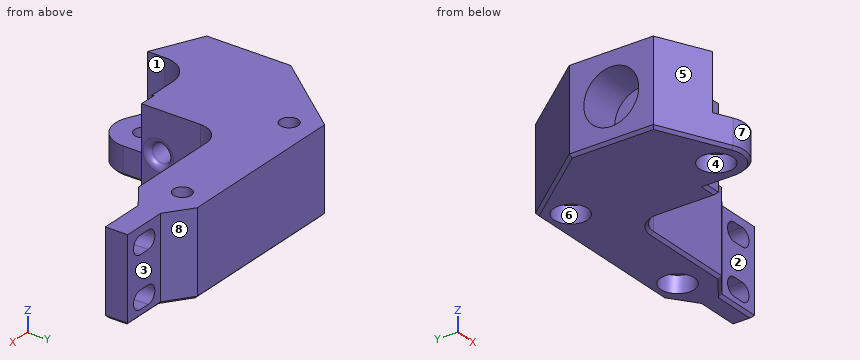
from build123d import *

# Parameters (mm, degrees)
BOX_W           = 10.4
BOX_H           = 10.4
BOX_DEPTH       = 10
CYLINDER_R      = 5.2
CYLINDER_DEPTH  = 10
BOX001_W        = 10.4
BOX001_H        = 10
BOX001_DEPTH    = 10
SKETCH001_R     = 1.6
PAD_DEPTH       = 20
SKETCH_R        = 3
PAD001_DEPTH    = 3
PAD002_DEPTH    = 15
SKETCH003_R     = 4.9
POCKET_DEPTH    = 7.5
SKETCH004_R     = 1.75
POCKET001_DEPTH = 47.501
POCKET002_DEPTH = 5
FILLET_R        = 4
FILLET001_R     = 1
CHAMFER_SIZE    = 0.5


with BuildPart() as cube:
    # Box → Box (new body)
    with BuildSketch(Plane(origin=(-13, -18.2, 5), x_dir=(1, 0, 0), z_dir=(0, 0, 1))):
        with Locations((5.2, 5.2)):
            Rectangle(BOX_W, BOX_H)
    extrude(amount=BOX_DEPTH)


with BuildPart() as cylinder:
    # Cylinder → Cylinder (new body)
    with BuildSketch(Plane(origin=(-13, -13, 5), x_dir=(1, 0, 0), z_dir=(0, 0, 1))):
        Circle(CYLINDER_R)
    extrude(amount=CYLINDER_DEPTH)


with BuildPart() as obj1:
    # Box001 → Box001 (new body)
    with BuildSketch(Plane(origin=(-18.2, -23, 5), x_dir=(1, 0, 0), z_dir=(0, 0, 1))):
        with Locations((5.2, 5)):
            Rectangle(BOX001_W, BOX001_H)
    extrude(amount=BOX001_DEPTH)

    # Fusion001: union Cube, Cylinder
    add(cube.part)
    add(cylinder.part)


with BuildPart() as cuerpo_tornillos:
    # Sketch001 → Pad (new body)
    with BuildSketch(Plane.XY.offset(3.25)):
        with Locations((-13, 13)):
            Circle(SKETCH001_R)
        with Locations((13, 13)):
            Circle(SKETCH001_R)
        with Locations((-13, -13)):
            Circle(SKETCH001_R)
    extrude(amount=PAD_DEPTH)


with BuildPart() as tornillos:
    # Sketch → Pad001 (new body)
    with BuildSketch(Plane.XY):
        with Locations((-13, 13)):
            Circle(SKETCH_R)
        with Locations((13, 13)):
            Circle(SKETCH_R)
        with Locations((-13, -13)):
            Circle(SKETCH_R)
    extrude(amount=PAD001_DEPTH)

    # Fusion: union cuerpo_tornillos
    add(cuerpo_tornillos.part)


with BuildPart() as chamfer_body:
    # Sketch002 → Pad002 (new body)
    with BuildSketch(Plane.XY):
        with BuildLine():
            Line((-15.109533, -17.533197), (-27, -12))
            Line((-27, -12), (-27, 3))
            Line((-27, 3), (-15.5, 17.5))
            Line((-15.5, 17.5), (15.5, 17.5))
            Line((15.5, 17.5), (20, 14.25))
            Line((20, 14.25), (28, 14.25))
            Line((28, 14.25), (28, 10.25))
            Line((28, 10.25), (20, 10.25))
            Line((20, 10.25), (15.5, 7))
            Line((15.5, 7), (-5, 7))
            Line((-5, 7), (-5, -7.5))
            Line((-5, -7.5), (-8, -7.5))
            Line((-8, -7.5), (-8, -13))
            ThreePointArc((-15.109533, -17.533197), (-10.311847, -17.215902), (-8, -13))
        make_face()
    extrude(amount=PAD002_DEPTH)

    # Sketch003 → Pocket (cut)
    with BuildSketch(Plane(origin=(-27, 0, 0), x_dir=(0, -1, 0), z_dir=(-1, 0, 0))):
        with Locations((4.5, 7.5)):
            Circle(SKETCH003_R)
    extrude(amount=-POCKET_DEPTH, mode=Mode.SUBTRACT)

    # Sketch004 → Pocket001 (cut, through all)
    with BuildSketch(Plane(origin=(-19.5, 0, 0), x_dir=(0, -1, 0), z_dir=(-1, 0, 0))):
        with Locations((4.5, 7.5)):
            Circle(SKETCH004_R)
    extrude(amount=-POCKET001_DEPTH, mode=Mode.SUBTRACT)

    # Sketch005 → Pocket002 (cut)
    with BuildSketch(Plane(origin=(0, 14.25, 0), x_dir=(-1, 0, 0), z_dir=(0, 1, 0))):
        with BuildLine():
            ThreePointArc((-25, 13.6), (-26.6, 12), (-25, 10.4))
            Line((-25, 10.4), (-23, 10.4))
            ThreePointArc((-23, 10.4), (-21.4, 12), (-23, 13.6))
            Line((-25, 13.6), (-23, 13.6))
        make_face()
        with BuildLine():
            ThreePointArc((-25, 4.6), (-26.6, 3), (-25, 1.4))
            Line((-25, 1.4), (-23, 1.4))
            ThreePointArc((-23, 1.4), (-21.4, 3), (-23, 4.6))
            Line((-25, 4.6), (-23, 4.6))
        make_face()
    extrude(amount=-POCKET002_DEPTH, mode=Mode.SUBTRACT)

    # Cut: cut tornillos
    add(tornillos.part, mode=Mode.SUBTRACT)

    # Cut001: cut obj1
    add(obj1.part, mode=Mode.SUBTRACT)

    # Fillet
    fillet_edges = [chamfer_body.edges().sort_by_distance(p)[0] for p in [
        (-5, 7, 7.5),
    ]]
    fillet(fillet_edges, radius=FILLET_R)

    # Fillet001
    fillet001_edges = [chamfer_body.edges().sort_by_distance(p)[0] for p in [
        (-5, -2.75, 7.5),
    ]]
    fillet(fillet001_edges, radius=FILLET001_R)

    # Chamfer
    chamfer_edges = [chamfer_body.edges().sort_by_distance(p)[0] for p in [
        (0, 17.5, 0),
        (-21.25, 10.25, 0),
        (-27, -4.5, 0),
        (-21.054766, -14.766598, 0),
        (-10.311847, -17.215902, 0),
        (-8, -10.25, 0),
        (-6.5, -7.5, 0),
        (-5, -2.25, 0),
        (-3.828427, 5.828427, 0),
        (7.25, 7, 0),
        (17.75, 8.625, 0),
        (24, 10.25, 0),
        (28, 12.25, 0),
        (24, 14.25, 0),
        (17.75, 15.875, 0),
    ]]
    chamfer(chamfer_edges, length=CHAMFER_SIZE)


solid = chamfer_body.part
Read the model definition and answer for the solid it produces. Units are mm, in the model's axes. Face numbers are marked on the shaded views. A direction names the side the tool comes from. Give positions to 0.01 mm unless a question says otherwise; leave off trailing zeros. Write each loop counter-clockwise with the first axis right and the second up, starting at its lowest first coordinate (ties: lowest second). Pieces come first, ordered by that corner, then holes. Notation, with made-up numbers: M 85,-17.75 L 96,-17.75 A23 ccw 96,13.25 Z; hole C 43.25,73.25 d10. An arc over 180 degrees is marked long. One line per item, written item: value. Start each with the question number.
(1) Determine the mould class of the marked faces 6, 7 and 8 for opening direction X: pulls with the +X half, pulls with the -X half, needs draft (parallel to the pull), parting line crosses it, or undercut.
(2) Find section D-D (x = 13). Determine the outline of the cut face in (y, z).
(3) Flat-ended cylindrical pins translate along their axes: pin 1 Ø3 at (y, z) = (-3.5, 6.5) entering from +X; pin 2 Ø5.5 at (x, y) = (-13, -13) entering from -Z; pin 3 Ø3 at (y, z) = (-4.5, 9.5) entering from -X; pin 4 Ø3 at (x, y) = (-2.5, -6.5) entering from -Z. Find the tip coordinate at first contact, or state that the pin passes through.
(4) Find section C-C (z = 11.25). Determine the outline of the cut face in (x, y), plus the area to 3 significant figures.
(5) A tool of negligible diameter and unlimited length cuts with its end or side. For the marked faces 1, 2, 3, 4 and 5, from which of +Z, -Z, +X, -X, +Y, -Y can it reach the whole face along a straight path? Write none if from no direction.
(6) Find the intervals of material crossed by line 1 (X direction, y = 13, z = 11.25); line 2 (X direction, y = -3.5, z = 10); line 3 (X direction, y = 13, z = 11), in increasing order.
(7) Find section B-B (x = 0.5). Determine the outline of the cut face in (y, z), plus the area to 3 significant figures.
(8) Find section A-A (z = 7.5). Give the number of separate pieces and of enclosed holes in the cut face, plus the area to 3 significant figures.
Results below:
1. face 6: undercut
1. face 7: parting line crosses it
1. face 8: pulls with the +X half
2. outline: M 7,0.5 L 7.5,0 L 10,0 L 10,3 L 16,3 L 16,0 L 17,0 L 17.5,0.5 L 17.5,15 L 14.6,15 L 14.6,3.25 L 11.4,3.25 L 11.4,15 L 7,15 Z
3. pin 1: stops at x = -5
3. pin 2: stops at z = 3
3. pin 3: stops at x = -19.5
3. pin 4: passes through
4. outline: M -27,-12 L -18.2,-16.1 L -18.2,-13 A5.2 cw -13,-7.8 L -8,-7.8 L -8,-7.5 L -5,-7.5 L -5,3 A4 cw -1,7 L 15.5,7 L 20,10.25 L 21.59,10.25 L 21.59,14.25 L 20,14.25 L 15.5,17.5 L -15.5,17.5 L -27,3 L -27,-1.35 L -19.5,-1.35 L -19.5,-7.65 L -27,-7.65 Z; M 26.41,10.25 L 28,10.25 L 28,14.25 L 26.41,14.25 Z; hole C -13,13 d3.2; hole C 13,13 d3.2
4. area: 734 mm^2
5. face 1: +Z, +X, -Y
5. face 2: +Z, -Z, +X, -Y
5. face 3: +Z, -Z, +X, +Y
5. face 4: -Z
5. face 5: +Z, -Z, -X, -Y
6. line 1: x = -19.07 to -14.6, -11.4 to 11.4, 14.6 to 21.59, 26.41 to 28
6. line 2: x = -19.5 to -5
6. line 3: x = -19.07 to -14.6, -11.4 to 11.4, 14.6 to 21.75, 26.25 to 28
7. outline: M 7,0.5 L 7.5,0 L 17,0 L 17.5,0.5 L 17.5,15 L 7,15 Z
7. area: 157 mm^2
8. separate pieces: 2
8. enclosed holes: 2
8. area: 676 mm^2
